```python
from build123d import *

# Parameters (mm, degrees)
SKETCH1_W           = 25.4
SKETCH1_H           = 25.4
SKETCH1_W_2         = 22.225
SKETCH1_H_2         = 22.225
BOSS_EXTRUDE1_DEPTH = 139.7
SKETCH2_R           = 1.984375
CUT_EXTRUDE1_DEPTH  = 26.4


with BuildPart() as part:
    # Sketch1 → Boss-Extrude1 (new body)
    with BuildSketch(Plane.XY):
        Rectangle(SKETCH1_W, SKETCH1_H)
        Rectangle(SKETCH1_W_2, SKETCH1_H_2, mode=Mode.SUBTRACT)
    extrude(amount=BOSS_EXTRUDE1_DEPTH)

    # Sketch2 → Cut-Extrude1 (cut, through all)
    with BuildSketch(Plane(origin=(0, 12.7, 0), x_dir=(1, 0, 0), z_dir=(0, 1, 0))):
        with Locations((0, -127)):
            Circle(SKETCH2_R)
        with Locations((0, -101.6)):
            Circle(SKETCH2_R)
        with Locations((0, -76.2)):
            Circle(SKETCH2_R)
        with Locations((0, -50.8)):
            Circle(SKETCH2_R)
        with Locations((0, -25.4)):
            Circle(SKETCH2_R)
        Circle(SKETCH2_R)
        with Locations((0, 25.4)):
            Circle(SKETCH2_R)
        with Locations((0, 50.8)):
            Circle(SKETCH2_R)
        with Locations((0, 76.2)):
            Circle(SKETCH2_R)
        with Locations((0, 101.6)):
            Circle(SKETCH2_R)
        with Locations((0, 127)):
            Circle(SKETCH2_R)
        with Locations((0, 152.4)):
            Circle(SKETCH2_R)
    extrude(amount=-CUT_EXTRUDE1_DEPTH, mode=Mode.SUBTRACT)


solid = part.part
```
Input: part model. Units: mm. Frame: model coordinates. A direction names the side the tool comes from. Round coordinates to 2 decimals unless told otherwise and drop trailing zeros. Loops run counter-clockwise (first coordinate to the right, second up) from the corner with the lowest first, then second, coordinate; pieces in that order, holes last.
1) Pull-direction query (Z, two-part tool) for faces 1 (the flat face through (-11.3, -0.9, 0)), 2 (the cylindrical face through (-0.43, 11.917, 103.537)), 3 (the flat face through (0, -11.112, 69)); classes: released by +Z, released by -Z, zero draft, split by the parting line, or undercut.
Ans:
face 1: released by -Z
face 2: undercut
face 3: zero draft
2) Set-up query: faces 4 (the flat face through (11.112, 0, 69)), 5 (the cylindrical face through (-0.43, 11.917, 52.737)). Return all of +Z, -Z, +X, -X, +Y, -Y with unobstructed straight access to the full face (end or side cutting, diameter ignored); none if empty.
Ans:
face 4: +Z, -Z
face 5: +Y, -Y
3) Material intervals for line 1 (Z direction, x = 0, y = -11.9); line 2 (X direction, y = 1.75, z = 85), sorted ascending.
Ans:
line 1: z = 1.98 to 23.42, 27.38 to 48.82, 52.78 to 74.22, 78.18 to 99.62, 103.58 to 125.02, 128.98 to 139.7
line 2: x = -12.7 to -11.11, 11.11 to 12.7
4) Section query C-C on z = 107.5. Return the cut outline in (x, y).
Ans:
outline: (-12.7, -12.7) - (12.7, -12.7) - (12.7, 12.7) - (-12.7, 12.7) - close; hole (-11.11, -11.11) - (11.11, -11.11) - (11.11, 11.11) - (-11.11, 11.11) - close
5) Section query A-A on y = -9.5. Return the cut outline in (x, z), plus the area to 3 significant figures.
Ans:
outline: (-12.7, 0) - (-11.11, 0) - (-11.11, 139.7) - (-12.7, 139.7) - close; (11.11, 0) - (12.7, 0) - (12.7, 139.7) - (11.11, 139.7) - close
area: 444 mm2
6) Section query D-D on x = 0. Count the separate pieces of the cut face and the enclosed holes in it, plus the area to 3 significant figures.
Ans:
separate pieces: 12
enclosed holes: 0
area: 374 mm2
